Read the model definition and answer for the solid it produces. Units are mm, in the model's axes. Face numbers are marked on the shaded views. A direction names the side the tool comes from. Give positions to 0.01 mm unless a question says otherwise; leave off trailing zeros. Write each loop counter-clockwise with the first axis right and the second up, starting at its lowest first coordinate (ties: lowest second). Pieces come first, ordered by that corner, then holes. Notation, with made-up numbers: (33, 44.25) -> (72, 44.25) arc R17 cw to (72, 69.25) -> close; hole circle Ø1 at (-26, 7). An arc over 180 degrees is marked (long way). Answer as CSV lines item,"result". Start each with the question number.
1. Find the intervals of material crossed by line 1 (Z direction, x = -47, y = 1); line 2 (X direction, y = 0.5, z = -1); line 3 (Y direction, x = 3.5, z = -12.5), in increasing order.
2. Given pin 1 (1.8 mm diameter, centred on x = -42.5, z = -7.5, fed in from +Y); pin 2 (2 mm diameter, centred on y = -3, z = -1, fed in from +X); pin 3 (6 mm diameter, centred on x = 1.5, z = -6, fed in from -Y); pin 4 (1.4 mm diameter, centred on x = -47, z = -1, fed in from -Y), each flat-ended and moving along its own axis, determine where each tip first touches the part or whether it passes through.
3. The part is cut by section B-B, the plane x = -1. Determine the outline of the cut face in (y, z).
4. For a pull along Z with two mould halves and no side action, classify the marked faces 1, 2 and 3 as pulls with the +Z half, pulls with the -Z half, needs draft (parallel to the pull), parting line crosses it, or undercut.
5. The part is cut by section C-C, the plane y = -3.5. Determine the outline of the cut face in (x, z).
6. The part is cut by section A-A, the plane z = -1. Determine the outline of the cut face in (x, y).
7. A tool of negligible diameter and unlimited length cuts with its end or side. For the marked faces 4, 5, 6, 7 and 8, from which of +Z, -Z, +X, -X, +Y, -Y can it reach the whole face along a straight path? Write none if from no direction.
8. The part is cut by section D-D, the plane z = -13.75. Determine the outline of the cut face in (x, y).
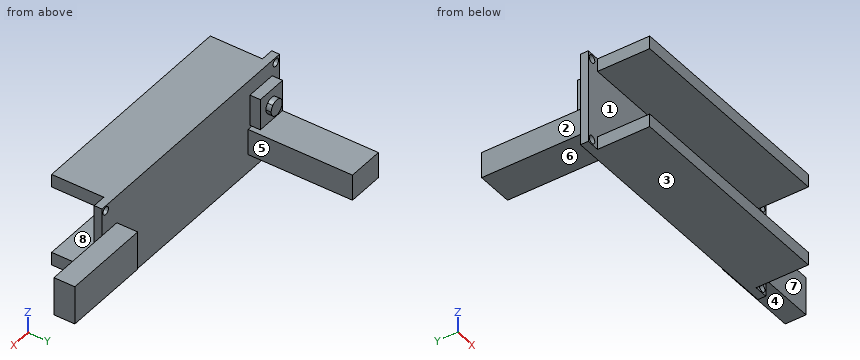
from build123d import *

# Parameters (mm, degrees)
SKETCH_1_W          = 48
SKETCH_1_H          = 18
EXTRUDE_1_DEPTH     = 1.5
EXTRUDE_2_DEPTH     = 4
SKETCH_4_W          = 42.9
SKETCH_4_H          = 2.5
EXTRUDE_3_DEPTH     = 10
SKETCH_5_W          = 7
SKETCH_5_H          = 5
EXTRUDE_4_DEPTH     = 20
SKETCH_6_W          = 6
SKETCH_6_H          = 6
EXTRUDE_5_DEPTH     = 2
EXTRUDE_6_DEPTH     = 1
SKETCH_8_R          = 0.75
CUT_EXTRUDE_1_DEPTH = 10


with BuildPart() as part:
    # Эскиз1 → Бобышка-Вытянуть1 (new body)
    with BuildSketch(Plane(origin=(0, 0, 0), x_dir=(1, 0, 0), z_dir=(0, 1, 0))):
        with Locations((-24, 9)):
            Rectangle(SKETCH_1_W, SKETCH_1_H)
    extrude(amount=EXTRUDE_1_DEPTH)

    # Эскиз2 → Бобышка-Вытянуть2 (add)
    with BuildSketch(Plane(origin=(0, 1.5, 0), x_dir=(1, 0, 0), z_dir=(0, 1, 0))):
        Polygon((0, 12.7), (0, 9), (0, 5.3), (13, 5.3), (13, 12.7), align=None)
        Polygon((0, 5.3), (0, 9), (0, 12.7), (-4, 12.7), (-4, 5.3), align=None)
    extrude(amount=EXTRUDE_2_DEPTH)

    # Эскиз4 → Бобышка-Вытянуть3 (add)
    with BuildSketch(Plane(origin=(0, 0, 0), x_dir=(-1, 0, 0), z_dir=(0, -1, 0))):
        with Locations((24.05, 16.75)):
            Rectangle(SKETCH_4_W, SKETCH_4_H)
        with Locations((24.05, 1.25)):
            Rectangle(SKETCH_4_W, SKETCH_4_H)
    extrude(amount=EXTRUDE_3_DEPTH)

    # Эскиз5 → Бобышка-Вытянуть4 (add)
    with BuildSketch(Plane(origin=(0, 1.5, 0), x_dir=(1, 0, 0), z_dir=(0, 1, 0))):
        with Locations((-43, 12)):
            Rectangle(SKETCH_5_W, SKETCH_5_H)
    extrude(amount=EXTRUDE_4_DEPTH)

    # Эскиз6 → Бобышка-Вытянуть5 (add)
    with BuildSketch(Plane(origin=(0, 1.5, 0), x_dir=(1, 0, 0), z_dir=(0, 1, 0))):
        with Locations((-43, 6)):
            Rectangle(SKETCH_6_W, SKETCH_6_H)
    extrude(amount=EXTRUDE_5_DEPTH)

    # Эскиз7 → Бобышка-Вытянуть6 (add)
    with BuildSketch(Plane(origin=(0, 3.5, 0), x_dir=(1, 0, 0), z_dir=(0, 1, 0))):
        with BuildLine():
            ThreePointArc((-41.939339828, 7.060660172), (-43, 7.5), (-44.060660172, 7.060660172))
            Line((-44.060660172, 7.060660172), (-43, 6))
            Line((-43, 6), (-41.939339828, 7.060660172))
        make_face()
        with BuildLine():
            Line((-43, 6), (-44.060660172, 7.060660172))
            ThreePointArc((-44.060660172, 7.060660172), (-44.5, 6), (-44.060660172, 4.939339828))
            Line((-44.060660172, 4.939339828), (-43, 6))
        make_face()
        with BuildLine():
            Line((-41.939339828, 7.060660172), (-43, 6))
            Line((-43, 6), (-41.939339828, 4.939339828))
            ThreePointArc((-41.939339828, 4.939339828), (-41.614180701, 5.425974851), (-41.5, 6))
            ThreePointArc((-41.5, 6), (-41.614180701, 6.574025149), (-41.939339828, 7.060660172))
        make_face()
        with BuildLine():
            Line((-41.939339828, 4.939339828), (-43, 6))
            Line((-43, 6), (-44.060660172, 4.939339828))
            ThreePointArc((-44.060660172, 4.939339828), (-43, 4.5), (-41.939339828, 4.939339828))
        make_face()
    extrude(amount=EXTRUDE_6_DEPTH)

    # Эскиз8 → Вырез-Вытянуть1 (cut)
    with BuildSketch(Plane(origin=(0, 1.5, 0), x_dir=(1, 0, 0), z_dir=(0, 1, 0))):
        with Locations(Location((-47, 17, 0), (0, 0, 270))):
            Circle(SKETCH_8_R)
        with Locations(Location((-47, 1, 0), (0, 0, 90))):
            Circle(SKETCH_8_R)
        with Locations(Location((-1, 1, 0), (0, 0, 270))):
            Circle(SKETCH_8_R)
        with Locations(Location((-1, 17, 0), (0, 0, 90))):
            Circle(SKETCH_8_R)
    extrude(amount=-CUT_EXTRUDE_1_DEPTH, mode=Mode.SUBTRACT)


solid = part.part
Results found:
1,line 1,"z = -18 to -17.75, -16.25 to -1.75, -0.25 to 0"
1,line 2,"x = -48 to -47.75, -46.25 to -1.75, -0.25 to 0"
1,line 3,"y = 1.5 to 5.5"
2,pin 1,"stops at y = 4.5"
2,pin 2,"stops at x = -2.6"
2,pin 3,"stops at y = 0"
2,pin 4,"passes through"
3,outline,"(0, -18) -> (1.5, -18) -> (1.5, -17.75) -> (0, -17.75) -> close; (0, -16.25) -> (1.5, -16.25) -> (1.5, -12.7) -> (5.5, -12.7) -> (5.5, -5.3) -> (1.5, -5.3) -> (1.5, -1.75) -> (0, -1.75) -> close; (0, -0.25) -> (1.5, -0.25) -> (1.5, 0) -> (0, 0) -> close"
4,face 1,"undercut"
4,face 2,"needs draft"
4,face 3,"pulls with the -Z half"
5,outline,"(-45.5, -18) -> (-2.6, -18) -> (-2.6, -15.5) -> (-45.5, -15.5) -> close; (-45.5, -2.5) -> (-2.6, -2.5) -> (-2.6, 0) -> (-45.5, 0) -> close"
6,outline,"(-48, 0) -> (-47.75, 0) -> (-47.75, 1.5) -> (-48, 1.5) -> close; (-46.25, 0) -> (-45.5, 0) -> (-45.5, -10) -> (-2.6, -10) -> (-2.6, 0) -> (-1.75, 0) -> (-1.75, 1.5) -> (-46.25, 1.5) -> close; (-0.25, 0) -> (0, 0) -> (0, 1.5) -> (-0.25, 1.5) -> close"
7,face 4,"-Z, +X, +Y"
7,face 5,"+Z, -Z, +Y"
7,face 6,"-Z, +X, -X, +Y"
7,face 7,"+Z, -Z, +X, -Y"
7,face 8,"+X, -X, -Y"
8,outline,"(-48, 0) -> (0, 0) -> (0, 1.5) -> (-39.5, 1.5) -> (-39.5, 21.5) -> (-46.5, 21.5) -> (-46.5, 1.5) -> (-48, 1.5) -> close"
